Model file for the job. Use its own axes, mm. A direction names the side the tool comes from. Round coordinates to 2 decimals unless told otherwise and drop trailing zeros. Loops run counter-clockwise (first coordinate to the right, second up) from the corner with the lowest first, then second, coordinate; pieces in that order, holes last. Notation, with made-up numbers: M 9,-11.5 L 68,-11.5 A37 ccw 68,27.5 Z; hole C -25,-12.5 d8. An arc over 180 degrees is marked long. Use a Markdown table: item, result. Add a question column.
Item 1: Pin check, flat tips, straight feed: P1, Ø4, axis at x = 29.5, z = -22.5, coming from the +Y side; P2, Ø5, axis at x = -33.5, y = 7, coming from the +Z side; P3, Ø1, axis at y = 9.5, z = -55, coming from the -X side. Stop position of each tip, or through.
Item 2: Saw through at B-B on x = 0. Write the cut outline in (y, z).
Item 3: Saw through at A-A on z = 0. Write the cut outline in (x, y), then the cut area to 3 significant figures.
Item 4: Wall check: L1, parallel to X at y = 13, z = 0; L2, parallel to X at y = 9, z = -28; L3, parallel to X at y = 24.5, z = 26.5. Give the ranges that are in metal, low to high. Write a range as from..to.
Item 5: Saw through at D-D on x = -25.5. Write the cut outline in (y, z), then the cut area to 3 significant figures.
Item 6: Saw through at C-C on y = 19.75. Write the cut outline in (x, z), then the cut area to 3 significant figures.
Item 7: Two-plate mould, pull along Z, no slides. Class faces 1 (the cylindrical face through (-80.54, 13.8, -17.88)), 2 (the flat face through (1, 0, 36)), 3 (the flat face through (31, 0.325, -23)): +Z half, -Z half, draft (parallel to the pull), parting line (faces both ways), or undercut.
Item 8: Tool access for faces 4 (the cylindrical face through (-21, 14, -28)), 5 (the cylindrical face through (35.457, 13.969, -25.516)): list every direction of +Z, -Z, +X, -X, +Y, -Y with a clear straight run to the whole face (end or side of a thin tool).
```python
from build123d import *

# Parameters (mm, degrees)
SKETCH1_R           = 82.5
BOSS_EXTRUDE1_DEPTH = 28
SKETCH2_R           = 35
CUT_EXTRUDE1_DEPTH  = 120.98541578
SKETCH3_R           = 8.020540442
CUT_EXTRUDE2_DEPTH  = 27.674716
CIRPATTERN1_START   = 0.325283743
CIRPATTERN1_DEPTH   = 27.674716257


# Read off the part's stored shape, not the designer's step: CirPattern1
with BuildPart() as part:
    # Sketch1 → Boss-Extrude1 (new body)
    with BuildSketch(Plane(origin=(0, 0, 0), x_dir=(1, 0, 0), z_dir=(0, 1, 0))):
        with Locations(Location((0, 0, 0), (0, 0, 270))):
            Circle(SKETCH1_R)
    extrude(amount=BOSS_EXTRUDE1_DEPTH)

    # Sketch2 → Cut-Extrude1 (cut, through all)
    with BuildSketch(Plane(origin=(0, 0, 0), x_dir=(1, 0, 0), z_dir=(0, 1, 0))):
        with Locations(Location((0, 0, 0), (0, 0, 270))):
            Circle(SKETCH2_R)
    extrude(amount=CUT_EXTRUDE1_DEPTH, mode=Mode.SUBTRACT)

    # Sketch3 → Cut-Extrude2 (cut)
    with BuildSketch(Plane(origin=(0, 28, 0), x_dir=(1, 0, 0), z_dir=(0, 1, 0))):
        with Locations((-35.665635629, 0)):
            Circle(SKETCH3_R)
    extrude(amount=-CUT_EXTRUDE2_DEPTH, mode=Mode.SUBTRACT)

    # CirPattern1 outline → CirPattern1 (cut)
    with BuildSketch(Plane(origin=(0, 0, 0), x_dir=(1, 0, 0), z_dir=(0, 1, 0)).offset(CIRPATTERN1_START)):
        with BuildLine():
            ThreePointArc((-3.056758429, -34.866262029), (-10.815594803, -33.28697807), (-18.020905107, -30.004116036))
            ThreePointArc((-18.020905107, -30.004116036), (-13.499770825, -41.548022424), (-3.056758429, -34.866262029))
        make_face()
        with BuildLine():
            ThreePointArc((-3.056758429, 34.866262029), (-13.499770825, 41.548022424), (-18.020905107, 30.004116036))
            ThreePointArc((-18.020905107, 30.004116036), (-10.815594803, 33.28697807), (-3.056758429, 34.866262029))
        make_face()
        with BuildLine():
            ThreePointArc((32.2151954, -13.68141752), (28.315594803, -20.57248383), (22.96684414, -26.410680988))
            ThreePointArc((22.96684414, -26.410680988), (35.34285886, -25.678090023), (32.2151954, -13.68141752))
        make_face()
        with BuildLine():
            ThreePointArc((32.2151954, 13.68141752), (35.34285886, 25.678090023), (22.96684414, 26.410680988))
            ThreePointArc((22.96684414, 26.410680988), (28.315594803, 20.57248383), (32.2151954, 13.68141752))
        make_face()
    extrude(amount=CIRPATTERN1_DEPTH, mode=Mode.SUBTRACT)


solid = part.part
```
Entries:
| question | item | result |
|---|---|---|
| 1 | P1 | y = 0.33 |
| 1 | P2 | z = 76.45 |
| 1 | P3 | x = -61.94 |
| 2 | outline | M 0,-82.5 L 28,-82.5 L 28,-35 L 0,-35 Z; M 0,35 L 28,35 L 28,82.5 L 0,82.5 Z |
| 3 | outline | M -82.5,0 L -35,0 L -35,0.33 L -43.69,0.33 L -43.69,28 L -82.5,28 Z; M 35,0 L 82.5,0 L 82.5,28 L 35,28 Z |
| 3 | area | 2,420 mm2 |
| 4 | L1 | -82.5..-43.69, 35..82.5 |
| 4 | L2 | -77.6..-21, 21..25, 32.7..77.6 |
| 4 | L3 | -78.13..-22.86, 22.86..23.05, 34.66..78.13 |
| 5 | outline | M 0,-78.46 L 28,-78.46 L 28,-23.97 L 0,-23.97 Z; M 0,23.97 L 28,23.97 L 28,78.46 L 0,78.46 Z |
| 5 | area | 3,050 mm2 |
| 6 | outline | C 0,0 d165; hole M -34.1,-7.87 A35 ccw -18.02,-30 A8.02 ccw long -3.06,-34.87 A35 ccw 22.97,-26.41 A8.02 ccw long 32.22,-13.68 A35 ccw 32.22,13.68 A8.02 ccw long 22.97,26.41 A35 ccw -3.06,34.87 A8.02 ccw long -18.02,30 A35 ccw -34.1,7.87 A8.02 ccw long Z |
| 6 | area | 17,000 mm2 |
| 7 | face 1 | parting line |
| 7 | face 2 | draft |
| 7 | face 3 | undercut |
| 8 | face 4 | +Y, -Y |
| 8 | face 5 | +Y |
